from build123d import *

# Parameters (mm, degrees)
SKETCH_W        = 50
SKETCH_H        = 15
PAD_DEPTH       = 3
SKETCH001_W     = 40
SKETCH001_H     = 15
PAD001_DEPTH    = 16
POCKET_DEPTH    = 30
SKETCH011_W     = 17
SKETCH011_H     = 15
POCKET001_DEPTH = 16
SKETCH004_R     = 2.75
HOLE_DEPTH      = 25
HOLE001_DEPTH   = 25
HOLE001_TIPS_R  = 2.75
POCKET002_DEPTH = 35
POCKET003_DEPTH = 5
SKETCH007_R     = 1.5
POCKET004_DEPTH = 10


with BuildPart() as part:
    # Sketch → Pad (new body)
    with BuildSketch(Plane.XY):
        Rectangle(SKETCH_W, SKETCH_H)
    extrude(amount=PAD_DEPTH)

    # Sketch001 (on Face6 of Pad) → Pad001 (join)
    with BuildSketch(Plane.XY.offset(3)):
        Rectangle(SKETCH001_W, SKETCH001_H)
    extrude(amount=PAD001_DEPTH)

    # Sketch002 (on Face9 of Pad001) → Pocket (cut)
    with BuildSketch(Plane.XZ.offset(7.5)):
        Polygon((-17.046261, 2.99842), (-13.147281, 19.007174), (-20.991112, 19.328264), (-20.991112, 2.99842), align=None)
        Polygon((17.046261, 2.99842), (13.147281, 19.007174), (20.991112, 19.328264), (20.991112, 2.99842), align=None)
    extrude(amount=-POCKET_DEPTH, mode=Mode.SUBTRACT)

    # Sketch011 (on Face11 of Pocket) → Pocket001 (cut)
    with BuildSketch(Plane.XY.offset(19)):
        Rectangle(SKETCH011_W, SKETCH011_H)
    extrude(amount=-POCKET001_DEPTH, mode=Mode.SUBTRACT)

    # Sketch004 → Hole (cut)
    with BuildSketch(Plane.YZ.offset(-8.5)):
        with Locations((0, 14.231076)):
            Circle(SKETCH004_R)
    extrude(amount=-HOLE_DEPTH, mode=Mode.SUBTRACT)

    # Sketch004 → Hole001 (cut)
    with BuildSketch(Plane.YZ.offset(-8.5)):
        with Locations((0, 14.231076)):
            Circle(SKETCH004_R)
    extrude(amount=HOLE001_DEPTH, mode=Mode.SUBTRACT)

    # Hole001 tips → Hole001 tip 1 section 0
    with BuildSketch(Plane.YZ.offset(16.5), mode=Mode.PRIVATE) as hole001_tip_1_s0:
        with Locations((0, 14.231076)):
            Circle(HOLE001_TIPS_R)
    loft([hole001_tip_1_s0.sketch, Vertex(18.152367, 0, 14.231076)], mode=Mode.SUBTRACT)

    # Sketch005 → Pocket002 (cut, symmetric)
    with BuildSketch(Plane(origin=(8.5, 0, 0), x_dir=(0, -1, 0), z_dir=(-1, 0, 0))):
        with BuildLine():
            ThreePointArc((-5.391307, 19.250991), (-6.817122, 18.478375), (-7.471648, 16.994637))
            Line((-7.471648, 16.994637), (-7.674281, 16.939731))
            Line((-7.674281, 16.939731), (-7.674281, 19.250991))
            Line((-5.391307, 19.250991), (-7.674281, 19.250991))
        make_face()
        with BuildLine():
            ThreePointArc((7.47165, 16.994637), (6.817123, 18.478376), (5.391307, 19.250992))
            Line((5.391307, 19.250992), (7.674281, 19.250992))
            Line((7.674281, 16.939731), (7.674281, 19.250992))
            Line((7.47165, 16.994637), (7.674281, 16.939731))
        make_face()
    extrude(amount=POCKET002_DEPTH, both=True, mode=Mode.SUBTRACT)

    # Sketch006 → Pocket003 (cut)
    with BuildSketch(Plane.XY.offset(3)):
        with BuildLine():
            ThreePointArc((-23.120269, 7.667623), (-24.453663, 7.11346), (-25.253739, 5.911415))
            Line((-25.253739, 5.911415), (-25.253739, 7.71409))
            Line((-25.253739, 7.71409), (-23.120269, 7.667623))
        make_face()
        with BuildLine():
            ThreePointArc((-25.38047, -5.775698), (-24.586864, -7.001599), (-23.25292, -7.595938))
            Line((-25.38047, -7.584312), (-23.25292, -7.595938))
            Line((-25.38047, -5.775698), (-25.38047, -7.584312))
        make_face()
        with BuildLine():
            ThreePointArc((25.253739, 5.911415), (24.453663, 7.113459), (23.12027, 7.667622))
            Line((25.253739, 7.71409), (23.12027, 7.667622))
            Line((25.253739, 5.911415), (25.253739, 7.71409))
        make_face()
        with BuildLine():
            ThreePointArc((23.25292, -7.595938), (24.586863, -7.001599), (25.380469, -5.775699))
            Line((25.380469, -5.775699), (25.380469, -7.584312))
            Line((25.380469, -7.584312), (23.25292, -7.595938))
        make_face()
    extrude(amount=-POCKET003_DEPTH, mode=Mode.SUBTRACT)

    # Sketch007 → Pocket004 (cut)
    with BuildSketch(Plane.XY.offset(3)):
        with Locations((-19.232222, 0)):
            Circle(SKETCH007_R)
        with Locations((19.232222, 0)):
            Circle(SKETCH007_R)
    extrude(amount=-POCKET004_DEPTH, mode=Mode.SUBTRACT)


solid = part.part
For this review, take the finished solid that the model builds, in its own axes (mm). A direction names the side the tool comes from. Round coordinates to 2 decimals unless told otherwise and drop trailing zeros. Write each loop counter-clockwise with the first axis right and the second up, starting at its lowest first coordinate (ties: lowest second). Pieces come first, ordered by that corner, then holes. Notation, with made-up numbers: (50, -34.5) - (71, -34.5) arc R21 cw to (71, -14.5) - close; hole circle Ø4 at (-33, 54). An arc over 180 degrees is marked (long way). Use a Markdown table: item, result.
Q1. We need section A-A (z = 13). Give the boundary of the cut face in (x, y).
Derived:
| item | result |
|---|---|
| outline | (-14.61, -7.5) - (-8.5, -7.5) - (-8.5, -2.46) - (-14.61, -2.46) - close; (-14.61, 2.46) - (-8.5, 2.46) - (-8.5, 7.5) - (-14.61, 7.5) - close; (8.5, -7.5) - (14.61, -7.5) - (14.61, -2.46) - (8.5, -2.46) - close; (8.5, 2.46) - (14.61, 2.46) - (14.61, 7.5) - (8.5, 7.5) - close |
Q2. Wall thickness on line 1 along Z through (x, y) = (12.75, 0); line 2 along X through (y, z) = (2.5, 17); line 3 along Y through (x, z) = (11, 14.75): over which ranges is each line inside the solid? List them lowest first.
Derived:
| item | result |
|---|---|
| line 1 | z = 0 to 11.48, 16.98 to 19 |
| line 2 | x = -13.64 to -8.5, 8.5 to 13.64 |
| line 3 | y = -7.5 to -2.7, 2.7 to 7.5 |
Q3. We need section C-C (y = 1). State how many separate pieces and enclosed holes the cut face has, plus the area to 3 significant figures.
Derived:
| item | result |
|---|---|
| separate pieces | 5 |
| enclosed holes | 0 |
| area | 288 mm2 |
Q4. Machinability: for faces 5 (the flat face through (-8.5, 0, 11)), 6 (the flat face through (-19, -2, 2.998)), 7 (the cylindrical face through (-24.475, 7.095, 1.521)), which of the approach directions +Z, -Z, +X, -X, +Y, -Y give a long, thin tool a straight path to every point of the face, cutting with its end or side? Answer none if there is none.
Derived:
| item | result |
|---|---|
| face 5 | +Z, +Y, -Y |
| face 6 | +Z, -X, +Y, -Y |
| face 7 | +Z, -Z, -X, +Y |
Q5. Clearance check with flat-ended pins moving along their axes: pin 1 (2.5 mm diameter, centred on x = 19.23, y = 0, fed in from +Z); pin 2 (8 mm diameter, centred on y = -4, z = 9, fed in from -X); pin 3 (5 mm diameter, centred on x = 14, y = 4.5, fed in from +Z); pin 4 (7.5 mm diameter, centred on x = 2.5, y = 1.5, fed in from +Z). State where each tip first meets the part, or that it passes through.
Derived:
| item | result |
|---|---|
| pin 1 | passes through |
| pin 2 | stops at x = -16.56 |
| pin 3 | stops at z = 19 |
| pin 4 | stops at z = 3 |
Q6. The part is to be moulded in two halves that separate along Y. For faces 1 (the flat face through (-0.3, -7.5, 2.7)), 2 (the cylindrical face through (-11.761, -0.596, 11.546)), 3 (the cylindrical face through (11.105, 7.051, 18.183)), 4 (the flat face through (15.125, -0.105, 10.887)), say which applies: pulls with the +Y half, pulls with the -Y half, needs draft (parallel to the pull), parting line crosses it, or undercut.
Derived:
| item | result |
|---|---|
| face 1 | pulls with the -Y half |
| face 2 | undercut |
| face 3 | pulls with the +Y half |
| face 4 | needs draft |
Q7. We need section B-B (z = 11). Give the boundary of the cut face in (x, y), plus the area to 3 significant figures.
Derived:
| item | result |
|---|---|
| outline | (-15.1, -7.5) - (-8.5, -7.5) - (-8.5, 7.5) - (-15.1, 7.5) - close; (8.5, -7.5) - (15.1, -7.5) - (15.1, 7.5) - (8.5, 7.5) - close |
| area | 198 mm2 |
